Part model, mm, in its own coordinate system. A direction names the side the tool comes from. Round coordinates to 2 decimals unless told otherwise and drop trailing zeros. Loops run counter-clockwise (first coordinate to the right, second up) from the corner with the lowest first, then second, coordinate; pieces in that order, holes last.
1) Probe line 1 (X direction, y = -5.5, z = 9.5); line 2 (Y direction, x = 0.75, z = 29); line 3 (X direction, y = -3, z = 19). List the from-to ranges inside material, lowest first.
2) Band-saw the part on B-B, the plane x = 0. Write the cut outline in (y, z), then the cut area to 3 significant figures.
3) Band-saw the part on C-C, the plane z = 29.5. Write the cut outline in (x, y), then the cut area to 3 significant figures.
4) Mould opens along X. For faces 5 (the flat face through (-1.5, -6, 12)), 6 (the flat face through (0, -2.5, 39.5)), 7 (the flat face through (0, -7, 12)) say: +X half, -X half, draft (parallel to the pull), parting line (faces both ways), or undercut.
5) Band-saw the part on D-D, the plane z = 22. Write the cut outline in (x, y).
6) Drop flat-ended pins along their axis: P1, Ø1.6, axis at x = 0.5, y = -3.5, coming from the +Z side; P2, Ø0.9, axis at y = 3.5, z = 33.5, coming from the -X side; P3, Ø0.7, axis at y = 5.5, z = 12, coming from the +X side. Give the stop position or say it passes through.
7) 3-axis set-ups, long thin cutter, end or side, ignore diameter. For faces 1 (the flat face through (1.5, -6, 12)), 2 (the flat face through (0, 4, 25)), 3 (the flat face through (-1.5, 6, 12)), 4 (the flat face through (1.5, -4, 32)): which of +Z, -Z, +X, -X, +Y, -Y reach the whole face in a straight line?
8) Band-saw the part on A-A, the plane z = 12. Write the cut outline in (x, y), then the cut area to 3 significant figures.
from build123d import *

# Parameters (mm, degrees)
F0_R         = 5
F1_DEPTH     = 5
F3_DEPTH     = 15
F5_DEPTH     = 5
F7_DEPTH     = 15
F8_T1_DEPTH  = 4.3413789951
F8_T3_DEPTH  = 3
F8_T5_DEPTH  = 4.3413789951
F8_T10_ANGLE = 204.0849815342
F8_T12_ANGLE = 204.0849815342
F8_T17_DEPTH = 6.913061983
F8_T21_DEPTH = 5.571682988
F8_T28_DEPTH = 6.913061983
F8_T32_DEPTH = 5.571682988
F8_T39_DEPTH = 6.913061983
F8_T43_DEPTH = 5.571682988
F8_T50_DEPTH = 5.571682988
F8_T54_DEPTH = 6.913061983


# Not quite as in the source:
# - a fillet or chamfer that OpenCascade refuses, or shapes differently, is made with other operations: its cross-section is extruded or revolved along the edge and cut away or added


with BuildPart() as f1:
    # F0 (on Top) → F1 (new body)
    with BuildSketch(Plane.XY):
        Circle(F0_R)
    extrude(amount=F1_DEPTH)

    # F2 (on face) → F3 (join)
    with BuildSketch(Plane.XY.offset(5)):
        with BuildLine():
            Line((-1.5, 7), (-1.5, 4.7696960071))
            ThreePointArc((-1.5, 4.7696960071), (-5, 0), (-1.5, -4.7696960071))
            Line((-1.5, -4.7696960071), (-1.5, -7))
            Line((-1.5, -7), (1.5, -7))
            Line((1.5, -7), (1.5, -4.7696960071))
            ThreePointArc((1.5, -4.7696960071), (5, 0), (1.5, 4.7696960071))
            Line((1.5, 4.7696960071), (1.5, 7))
            Line((1.5, 7), (-1.5, 7))
        make_face()
    extrude(amount=F3_DEPTH)

    # F4 (on face) → F5 (join)
    with BuildSketch(Plane.XY.offset(20)):
        with BuildLine():
            ThreePointArc((1.5, -4.7696960071), (4.0311288741, -2.9580398915), (5, 0))
            ThreePointArc((5, 0), (4.0311288741, 2.9580398915), (1.5, 4.7696960071))
            ThreePointArc((1.5, 4.7696960071), (0, 5), (-1.5, 4.7696960071))
            ThreePointArc((-1.5, 4.7696960071), (-5, 0), (-1.5, -4.7696960071))
            ThreePointArc((-1.5, -4.7696960071), (0, -5), (1.5, -4.7696960071))
        make_face()
    extrude(amount=F5_DEPTH)

    # F6 (on face) → F7 (join)
    with BuildSketch(Plane.XY.offset(25)):
        with BuildLine():
            Line((1.5, -3), (1.5, -4.7696960071))
            ThreePointArc((1.5, -4.7696960071), (5, 0), (1.5, 4.7696960071))
            Line((1.5, 4.7696960071), (1.5, 3))
            Line((1.5, 3), (-1.5, 3))
            Line((-1.5, 3), (-1.5, 4.7696960071))
            ThreePointArc((-1.5, 4.7696960071), (-5, 0), (-1.5, -4.7696960071))
            Line((-1.5, -4.7696960071), (-1.5, -3))
            Line((-1.5, -3), (1.5, -3))
        make_face()
    extrude(amount=F7_DEPTH)

    # F8: chamfer of 1 on 9 edges, made by hand

    # F8_s2 → F8_t1 (cut)
    with BuildSketch(Plane.XZ.offset(3)):
        Polygon((-2.5, 40), (-1.5, 39), (-1.5, 40), align=None)
        Polygon((1.5, 39), (2.5, 40), (1.5, 40), align=None)
    extrude(amount=F8_T1_DEPTH, mode=Mode.SUBTRACT)

    # F8_s4 → F8_t3 (cut)
    with BuildSketch(Plane.YZ.offset(-1.5)):
        Polygon((-2, 40), (-3, 39), (-3, 40), align=None)
        Polygon((2, 40), (3, 39), (3, 40), align=None)
    extrude(amount=F8_T3_DEPTH, mode=Mode.SUBTRACT)

    # F8_s6 → F8_t5 (cut)
    with BuildSketch(Plane.XZ.offset(-7.3413789951)):
        Polygon((1.5, 39), (2.5, 40), (1.5, 40), align=None)
        Polygon((-2.5, 40), (-1.5, 39), (-1.5, 40), align=None)
    extrude(amount=F8_T5_DEPTH, mode=Mode.SUBTRACT)

    # F8_s7 → F8_t8 (revolve, cut)
    with BuildSketch(Plane.XZ):
        Polygon((5, 1), (4, 0), (5, 0), align=None)
    revolve(axis=Axis((0, 0, 0), (0, 0, 1)), mode=Mode.SUBTRACT)

    # F8_s9 → F8_t10 (revolve, cut)
    with BuildSketch(Plane(origin=(0, 0, 0), x_dir=(0, 0, 1), z_dir=(-0.9779931437, 0.2086370315, 0))):
        Polygon((39, -5), (40, -4), (40, -5), align=None)
    revolve(axis=Axis((0, 0, 40), (0, 0, 1)), revolution_arc=F8_T10_ANGLE, mode=Mode.SUBTRACT)

    # F8_s11 → F8_t12 (revolve, cut)
    with BuildSketch(Plane(origin=(0, 0, 0), x_dir=(0, 0, 1), z_dir=(0.9779931437, -0.2086370315, 0))):
        Polygon((39, -5), (40, -4), (40, -5), align=None)
    revolve(axis=Axis((0, 0, 40), (0, 0, 1)), revolution_arc=F8_T12_ANGLE, mode=Mode.SUBTRACT)


with BuildPart() as f8_tool15:
    # F8_s16 → F8_t17 (new body)
    with BuildSketch(Plane.XZ.offset(7.3413789951)):
        Polygon((-2.5, 40), (-1.5, 39), (-1.5, 40), align=None)
    extrude(amount=-F8_T17_DEPTH)

    split(bisect_by=Plane.XZ.offset(3), keep=Keep.BOTTOM)


with BuildPart() as f8_tool19:
    # F8_s20 → F8_t21 (new body)
    with BuildSketch(Plane.YZ.offset(-4.071682988)):
        Polygon((-2, 40), (-3, 39), (-3, 40), align=None)
    extrude(amount=F8_T21_DEPTH)

    split(bisect_by=Plane.YZ.offset(-1.5), keep=Keep.BOTTOM)


with BuildPart() as f8_tool15_1:
    add(f8_tool15.part)

    # F8_t23: intersect F8_tool19
    add(f8_tool19.part, mode=Mode.INTERSECT)


with BuildPart() as f1_1:
    add(f1.part)

    # F8_t13: cut F8_tool15
    add(f8_tool15_1.part, mode=Mode.SUBTRACT)


with BuildPart() as f8_tool26:
    # F8_s27 → F8_t28 (new body)
    with BuildSketch(Plane.XZ.offset(0.428317012)):
        Polygon((1.5, 39), (2.5, 40), (1.5, 40), align=None)
    extrude(amount=F8_T28_DEPTH)

    split(bisect_by=Plane.XZ.offset(3), keep=Keep.BOTTOM)


with BuildPart() as f8_tool30:
    # F8_s31 → F8_t32 (new body)
    with BuildSketch(Plane.YZ.offset(-1.5)):
        Polygon((-2, 40), (-3, 39), (-3, 40), align=None)
    extrude(amount=F8_T32_DEPTH)

    split(bisect_by=Plane.YZ.offset(1.5), keep=Keep.TOP)


with BuildPart() as f8_tool26_1:
    add(f8_tool26.part)

    # F8_t34: intersect F8_tool30
    add(f8_tool30.part, mode=Mode.INTERSECT)


with BuildPart() as f1_2:
    add(f1_1.part)

    # F8_t24: cut F8_tool26
    add(f8_tool26_1.part, mode=Mode.SUBTRACT)


with BuildPart() as f8_tool37:
    # F8_s38 → F8_t39 (new body)
    with BuildSketch(Plane.XZ.offset(-7.3413789951)):
        Polygon((1.5, 39), (2.5, 40), (1.5, 40), align=None)
    extrude(amount=F8_T39_DEPTH)

    split(bisect_by=Plane.XZ.offset(-3), keep=Keep.TOP)


with BuildPart() as f8_tool41:
    # F8_s42 → F8_t43 (new body)
    with BuildSketch(Plane.YZ.offset(4.071682988)):
        Polygon((2, 40), (3, 39), (3, 40), align=None)
    extrude(amount=-F8_T43_DEPTH)

    split(bisect_by=Plane.YZ.offset(1.5), keep=Keep.TOP)


with BuildPart() as f8_tool37_1:
    add(f8_tool37.part)

    # F8_t45: intersect F8_tool41
    add(f8_tool41.part, mode=Mode.INTERSECT)


with BuildPart() as f1_3:
    add(f1_2.part)

    # F8_t35: cut F8_tool37
    add(f8_tool37_1.part, mode=Mode.SUBTRACT)


with BuildPart() as f8_tool48:
    # F8_s49 → F8_t50 (new body)
    with BuildSketch(Plane.YZ.offset(1.5)):
        Polygon((2, 40), (3, 39), (3, 40), align=None)
    extrude(amount=-F8_T50_DEPTH)

    split(bisect_by=Plane.YZ.offset(-1.5), keep=Keep.BOTTOM)


with BuildPart() as f8_tool52:
    # F8_s53 → F8_t54 (new body)
    with BuildSketch(Plane.XZ.offset(-0.428317012)):
        Polygon((-2.5, 40), (-1.5, 39), (-1.5, 40), align=None)
    extrude(amount=-F8_T54_DEPTH)

    split(bisect_by=Plane.XZ.offset(-3), keep=Keep.TOP)


with BuildPart() as f8_tool48_1:
    add(f8_tool48.part)

    # F8_t56: intersect F8_tool52
    add(f8_tool52.part, mode=Mode.INTERSECT)


with BuildPart() as f1_4:
    add(f1_3.part)

    # F8_t46: cut F8_tool48
    add(f8_tool48_1.part, mode=Mode.SUBTRACT)


solid = f1_4.part
Reported:
1. line 1: x = -1.5 to 1.5
1. line 2: y = -3 to 3
1. line 3: x = -4 to 4
2. outline: (-7, 5) - (-5, 5) - (-5, 1) - (-4, 0) - (4, 0) - (5, 1) - (5, 5) - (7, 5) - (7, 20) - (5, 20) - (5, 25) - (3, 25) - (3, 39) - (2, 40) - (-2, 40) - (-3, 39) - (-3, 25) - (-5, 25) - (-5, 20) - (-7, 20) - close
2. area: 398 mm2
3. outline: (-1.5, -4.77) - (-1.5, -3) - (1.5, -3) - (1.5, -4.77) arc R5 ccw to (1.5, 4.77) - (1.5, 3) - (-1.5, 3) - (-1.5, 4.77) arc R5 ccw to start
3. area: 67.0 mm2
4. face 5: -X half
4. face 6: undercut
4. face 7: draft
5. outline: circle Ø10 at (0, 0)
6. P1: stops at z = 39.3
6. P2: stops at x = -3.96
6. P3: stops at x = 1.5
7. face 1: +Z, -Z, +X, -Y
7. face 2: +Z, +Y
7. face 3: +Z, -Z, -X, +Y
7. face 4: +Z, -Y
8. outline: (-1.5, -7) - (1.5, -7) - (1.5, -4.77) arc R5 ccw to (1.5, 4.77) - (1.5, 7) - (-1.5, 7) - (-1.5, 4.77) arc R5 ccw to (-1.5, -4.77) - close
8. area: 91.0 mm2
